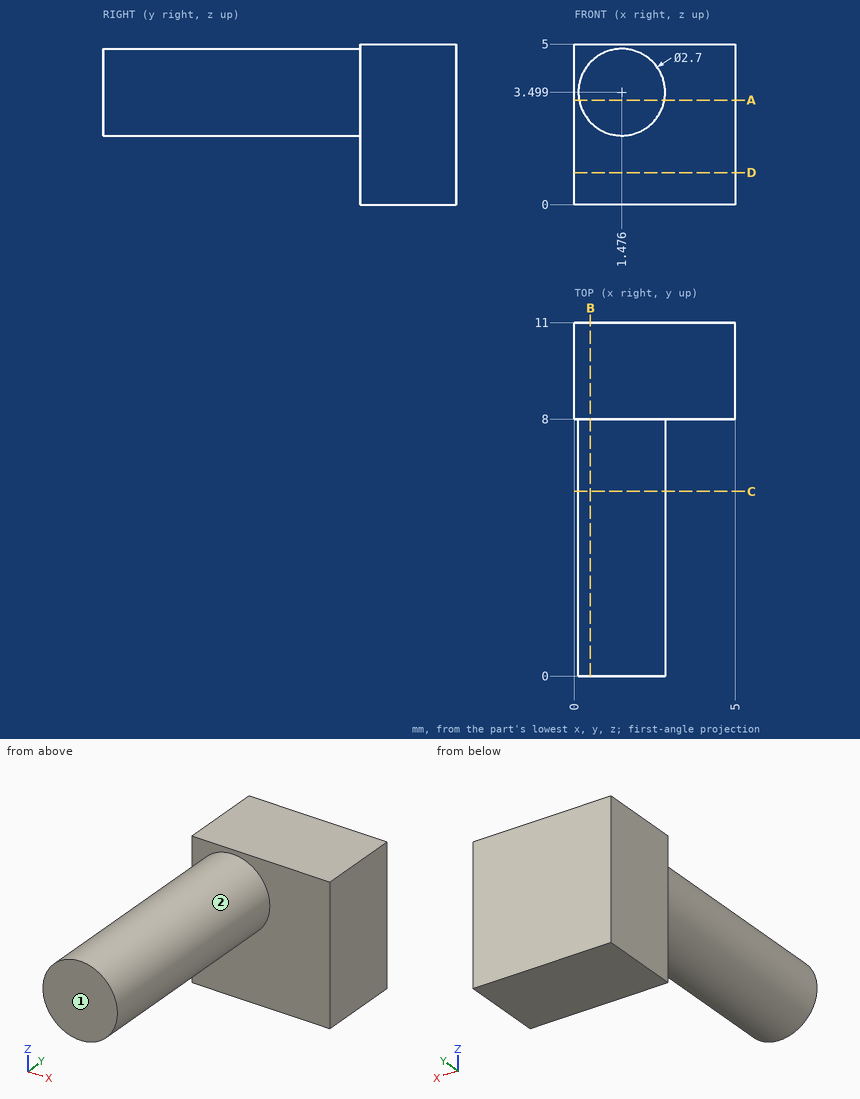
Geometry check sheet. Reference: drawing and pictorial views, mm from the part's lowest x, y, z. A direction names the side the tool comes from. Give positions to 0.01 mm unless a question says otherwise; leave off trailing zeros. Order: outer loops, then holes, each group sorted by start corner. A loop starts at its lowest first (then second) coordinate and runs counter-clockwise, first axis right, second up. Notation, with made-up numbers: M 80,63.5 L 94,63.5 A16 ccw 94,68.5 Z; hole C 40.5,-28 d8. An arc over 180 degrees is marked long. Answer as a JSON object with one key per item and string values. Group by question number.
1) Access from +Z, -Z, +X, -X, +Y, -Y to the whole of each face (thin tool, end or side, straight path). Record for the marked faces 1 and 2.
2) Cross-section at D-D (z = 1). Enter the section's corners in (x, y).
3) Cross-section at B-B (x = 0.5). Enter the section's corners in (y, z).
4) Depth check by flat-ended pin: pin 1 Ø3 at (y, z) = (5, 4.5) entering from +X; pin 2 Ø3 at (y, z) = (4.5, 2.5) entering from -X. Enter the tip coordinate at first touch or a pass-through.
5) Cross-section at C-C (y = 5.75). Enter the section's corners in (x, z).
6) Scan lines: line 1 along Y through (x, z) = (3, 4.5); line 2 along Z through (x, y) = (2.2, 4.5); line 3 along Z through (x, y) = (2.35, 6). Record each from-to range of solid material in increasing order. Write a range as [from, to].
7) Cross-section at A-A (z = 3.25). Enter the section's corners in (x, y), then the cut area to 3 significant figures.
Result sheet:
{
 "1": {"face 1": "+Z, -Z, +X, -X, -Y", "face 2": "-Y"},
 "2": {"outline": "M 0,8 L 5,8 L 5,11 L 0,11 Z"},
 "3": {"outline": "M 0,2.57 L 8,2.57 L 8,0 L 11,0 L 11,5 L 8,5 L 8,4.43 L 0,4.43 Z"},
 "4": {"pin 1": "stops at x = 2.83", "pin 2": "stops at x = 0.13"},
 "5": {"outline": "C 1.48,3.5 d2.7"},
 "6": {"line 1": "y = [8, 11]", "line 2": "z = [2.36, 4.64]", "line 3": "z = [2.47, 4.53]"},
 "7": {"outline": "M 0,8 L 0.15,8 L 0.15,0 L 2.8,0 L 2.8,8 L 5,8 L 5,11 L 0,11 Z", "area": "36.2 mm2"}
}
